CAD build for the part. Positions are in the model's coordinates, mm. A direction names the side the tool comes from. Round coordinates to 2 decimals unless told otherwise and drop trailing zeros. Order: outer loops, then holes, each group sorted by start corner. A loop starts at its lowest first (then second) coordinate and runs counter-clockwise, first axis right, second up. Notation, with made-up numbers: M 81.25,72.25 L 121.25,72.25 A9 ccw 121.25,80.25 Z; hole C 27,0 d9. An arc over 180 degrees is marked long. Answer as a JSON object with one key per item and string values.
```python
from build123d import *

# Parameters (mm, degrees)
F1_DEPTH = 36
F2_R     = 2.2
F4_DEPTH = 3.001
F3_R     = 2.2
F5_DEPTH = 10.7144513162
F3_R_2   = 3
F6_DEPTH = 1
F2_R_2   = 3
F7_DEPTH = 1


with BuildPart() as f1:
    # F0 (on Front) → F1 (new body)
    with BuildSketch(Plane.XZ):
        Polygon((0, 24), (0, 0), (22.5526228989, -8.2084834398), (23.3320459743, -5.2996369217), (3, 2.1006226146), (3, 24), align=None)
    extrude(amount=F1_DEPTH)

    # F2 (on face) → F4 (cut, through all)
    with BuildSketch(Plane.YZ.offset(3)):
        with Locations((-27, 19.0503113073)):
            Circle(F2_R)
        with Locations((-27, 7.0503113073)):
            Circle(F2_R)
        with Locations((-9, 7.0503113073)):
            Circle(F2_R)
        with Locations((-9, 19.0503113073)):
            Circle(F2_R)
    extrude(amount=-F4_DEPTH, mode=Mode.SUBTRACT)

    # F3 (on face) → F5 (cut, through all)
    with BuildSketch(Plane(origin=(1.02606043, 0, 2.8190778624), x_dir=(0.9396926208, 0, -0.3420201433), z_dir=(0.3420201433, 0, 0.9396926208))):
        with Locations((6.919078312, -27)):
            Circle(F3_R)
        with Locations((18.919078312, -27)):
            Circle(F3_R)
        with Locations((6.919078312, -9)):
            Circle(F3_R)
        with Locations((18.919078312, -9)):
            Circle(F3_R)
    extrude(amount=-F5_DEPTH, mode=Mode.SUBTRACT)

    # F3 (on face) → F6 (cut)
    with BuildSketch(Plane(origin=(1.02606043, 0, 2.8190778624), x_dir=(0.9396926208, 0, -0.3420201433), z_dir=(0.3420201433, 0, 0.9396926208))):
        with Locations((6.919078312, -27)):
            Circle(F3_R_2)
        with Locations((6.919078312, -27)):
            Circle(F3_R, mode=Mode.SUBTRACT)
        with Locations((18.919078312, -27)):
            Circle(F3_R_2)
        with Locations((18.919078312, -27)):
            Circle(F3_R, mode=Mode.SUBTRACT)
        with Locations((18.919078312, -9)):
            Circle(F3_R_2)
        with Locations((18.919078312, -9)):
            Circle(F3_R, mode=Mode.SUBTRACT)
        with Locations((6.919078312, -9)):
            Circle(F3_R_2)
        with Locations((6.919078312, -9)):
            Circle(F3_R, mode=Mode.SUBTRACT)
    extrude(amount=-F6_DEPTH, mode=Mode.SUBTRACT)

    # F2 (on face) → F7 (cut)
    with BuildSketch(Plane.YZ.offset(3)):
        with Locations((-27, 19.0503113073)):
            Circle(F2_R_2)
        with Locations((-27, 19.0503113073)):
            Circle(F2_R, mode=Mode.SUBTRACT)
        with Locations((-9, 7.0503113073)):
            Circle(F2_R_2)
        with Locations((-9, 7.0503113073)):
            Circle(F2_R, mode=Mode.SUBTRACT)
        with Locations((-9, 19.0503113073)):
            Circle(F2_R_2)
        with Locations((-9, 19.0503113073)):
            Circle(F2_R, mode=Mode.SUBTRACT)
        with Locations((-27, 7.0503113073)):
            Circle(F2_R_2)
        with Locations((-27, 7.0503113073)):
            Circle(F2_R, mode=Mode.SUBTRACT)
    extrude(amount=-F7_DEPTH, mode=Mode.SUBTRACT)


solid = f1.part
```
Item 1: Wall check: line 1 along Y through (x, z) = (1, 21); line 2 along Z through (x, y) = (2.2, -9); line 3 along Z through (x, y) = (2.35, -9). Give the ranges that are in metal, low to high. Write a range as [from, to].
Worked answers:
{"line 1": "y = [-36, -28.02], [-25.98, -10.02], [-7.98, 0]", "line 2": "z = [-0.8, 4.05], [10.05, 16.05], [22.05, 24]", "line 3": "z = [-0.86, 4.05], [10.05, 16.05], [22.05, 24]"}
Item 2: Drop flat-ended pins along their axis: pin 1 Ø2.5 at (y, z) = (-27, 19.05) entering from -X (3 decimals); pin 2 Ø5 at (y, z) = (-9, 19.05) entering from +X; pin 3 Ø5 at (y, z) = (-7, -1) entering from +X; pin 4 Ø2 at (x, y) = (9.5, -30) entering from +Z. Give the stop position or say it passes through.
Worked answers:
{"pin 1": "passes through", "pin 2": "stops at x = 2", "pin 3": "stops at x = 17.96", "pin 4": "stops at z = 0.1"}
Item 3: Saw through at A-A on y = -21. List the corners of the cut face in (x, z).
Worked answers:
{"outline": "M 0,0 L 22.55,-8.21 L 23.33,-5.3 L 3,2.1 L 3,24 L 0,24 Z"}
Item 4: Saw through at B-B on z = 15. List the corners of the cut face in (x, y).
Worked answers:
{"outline": "M 0,-36 L 3,-36 L 3,0 L 0,0 Z"}
Item 5: Saw through at C-C on y = -27. State how many separate pieces and enclosed holes the cut face has, and give its area (3 significant figures).
Worked answers:
{"separate pieces": "5", "enclosed holes": "0", "area": "78.1 mm2"}
Item 6: 3-axis set-ups, long thin cutter, end or side, ignore diameter. For faces 1 (the flat face through (22.94, -17.75, -6.77)), 2 (the flat face through (3, -18, 13)), 3 (the flat face through (2, -11, 9)): which of +Z, -Z, +X, -X, +Y, -Y reach the whole face in a straight line?
Worked answers:
{"face 1": "-Z, +X, +Y, -Y", "face 2": "+Z, +X, +Y, -Y", "face 3": "+X"}
Item 7: Two-plate mould, pull along X, no slides. Class faces 4 (the flat face through (13.31, -17.75, -1.65)), 5 (the cylindrical face through (17.86, -6.82, -5.42)), 6 (the cylindrical face through (2.507, -9.391, 22.025)): released by +X, released by -X, zero draft, split by the parting line, or undercut.
Worked answers:
{"face 4": "released by +X", "face 5": "undercut", "face 6": "zero draft"}
